Part model, mm, in its own coordinate system. Face numbers are marked on the shaded views. A direction names the side the tool comes from. Coordinates: 2 decimals unless noted, no trailing zeros. Order: outer loops, then holes, each group sorted by start corner. A loop starts at its lowest first (then second) coordinate and runs counter-clockwise, first axis right, second up.
1) Cut at A-A (z = 0). List the corners of the cut face in (x, y).
2) Cut at D-D (x = 13.75). List the corners of the cut face in (y, z).
3) Mould opens along X. For the marked faces 1, 2 and 3 say: +X half, -X half, draft (parallel to the pull), parting line (faces both ways), or undercut.
4) Cut at B-B (y = 0). List the corners of the cut face in (x, z), and give its area (3 significant figures).
5) Cut at C-C (x = 3.25). List the corners of the cut face in (y, z).
6) Tool access for the marked faces 4 and 5: list every direction of +Z, -Z, +X, -X, +Y, -Y with a clear straight run to the whole face (end or side of a thin tool).
7) Pin check, flat tips, straight feed: pin 1 Ø2 at (x, z) = (14, -5) entering from -Y; pin 2 Ø2 at (x, z) = (9.5, -1) entering from -Y; pin 3 Ø4.5 at (y, z) = (1, 0) entering from +X. Stop position of each tip, or through.
8) Wall check: L1, parallel to X at y = 0.75, z = 5.5; L2, parallel to X at y = -0.75, z = -2; L3, parallel to Z at x = 5.25, y = -0.25. Give the ranges that are in metal, low to high.
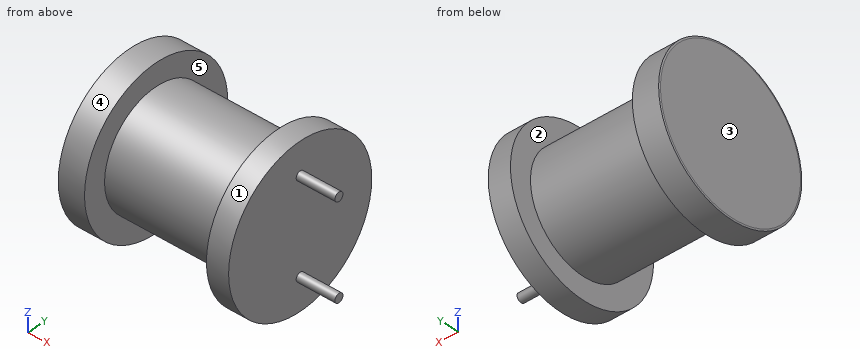
```python
from build123d import *

# Parameters (mm, degrees)
SKETCH_2_R      = 0.4
EXTRUDE_1_DEPTH = 3.5


with BuildPart() as part:
    # Эскиз1 → Повернуть1 (revolve)
    with BuildSketch(Plane.XY):
        Polygon((0, 0), (0, 7), (0.031301632, 7.15), (2.4, 7.15), (2.4, 5.15), (13.4, 5.15), (13.4, 7.15), (15.4, 7.15), (15.4, 0), align=None)
    revolve(axis=Axis((-29.538793103, 0, 0), (1, 0, 0)))

    # Эскиз2 → Бобышка-Вытянуть1 (add)
    with BuildSketch(Plane(origin=(15.4, 0, 0), x_dir=(0, 0, -1), z_dir=(1, 0, 0))):
        with Locations((-4.25, 0)):
            Circle(SKETCH_2_R)
        with Locations((4.25, 0)):
            Circle(SKETCH_2_R)
    extrude(amount=EXTRUDE_1_DEPTH)


solid = part.part
```
Geometry check:
1. outline: (0, -7) - (0.03, -7.15) - (2.4, -7.15) - (2.4, -5.15) - (13.4, -5.15) - (13.4, -7.15) - (15.4, -7.15) - (15.4, 7.15) - (13.4, 7.15) - (13.4, 5.15) - (2.4, 5.15) - (2.4, 7.15) - (0.03, 7.15) - (0, 7) - close
2. outline: circle Ø14.3 at (0, 0)
3. face 1: draft
3. face 2: undercut
3. face 3: -X half
4. outline: (0, -7) - (0.03, -7.15) - (2.4, -7.15) - (2.4, -5.15) - (13.4, -5.15) - (13.4, -7.15) - (15.4, -7.15) - (15.4, -4.65) - (18.9, -4.65) - (18.9, -3.85) - (15.4, -3.85) - (15.4, 3.85) - (18.9, 3.85) - (18.9, 4.65) - (15.4, 4.65) - (15.4, 7.15) - (13.4, 7.15) - (13.4, 5.15) - (2.4, 5.15) - (2.4, 7.15) - (0.03, 7.15) - (0, 7) - close
4. area: 182 mm2
5. outline: circle Ø10.3 at (0, 0)
6. face 4: +X, -X
6. face 5: none
7. pin 1: stops at y = -5.93
7. pin 2: stops at y = -5.15
7. pin 3: stops at x = 15.4
8. L1: x = 0 to 2.4, 13.4 to 15.4
8. L2: x = 0 to 15.4
8. L3: z = -5.14 to 5.14
